Here's the drawing with two shaded views (mm, measured from the low corner). I have some questions. A direction names the side the tool comes from. Give positions to 0.01 mm unless a question says otherwise; leave off trailing zeros. Loops run counter-clockwise (first coordinate to the right, second up) from the corner with the lowest first, then second, coordinate; pieces in that order, holes last. Notation, with made-up numbers: M -16,45 L -10,45 A27 cw -10,71 Z; hole C 76,-1 d5. An arc over 180 degrees is marked long. Use a Markdown table: item, result. Add a question column.
1) Suppose I cut it at D-D on x = 72.5. List the corners of the cut face in (y, z) for me, and give its area (3 significant figures).
2) Suppose I cut it at A-A on z = 2. List the corners of the cut face in (x, y) for me.
3) If I drill on line 1 along Y through (x, z) = (45.5, 3); line 2 along X through (y, z) = (9, 5); line 3 along Y through (x, z) = (74.5, 4.25), over which ranges is the centre line in solid material (lowest first)? Write a range as [from, to].
4) We'd pull the mould along X, two halves only. Please class the marked faces 6, 7, 8 and 9: +X half, -X half, draft (parallel to the pull), parting line (faces both ways), or undercut.
5) Suppose I cut it at B-B on y = 20. List the corners of the cut face in (x, z) for me, and give its area (3 significant figures).
6) Suppose I cut it at C-C on x = 45.5. List the corners of the cut face in (y, z) for me, and give its area (3 significant figures).
7) Will these pins go through, and if not, where does the flat tip stop? pin 1 Ø0.6 at (y, z) = (34.5, 2.5) entering from -X; pin 2 Ø4 at (x, z) = (15, 2) entering from -Y; pin 3 Ø0.6 at (y, z) = (33.5, 4) entering from +X; pin 4 Ø2 at (x, y) = (72, 5.5) entering from +Z.
8) Which directions (+Z, -Z, +X, -X, +Y, -Y) give clear straight access to the entire face, cutting with the end or side of a thin tool? Please do the marked faces 1, 2, 3, 4 and 5.
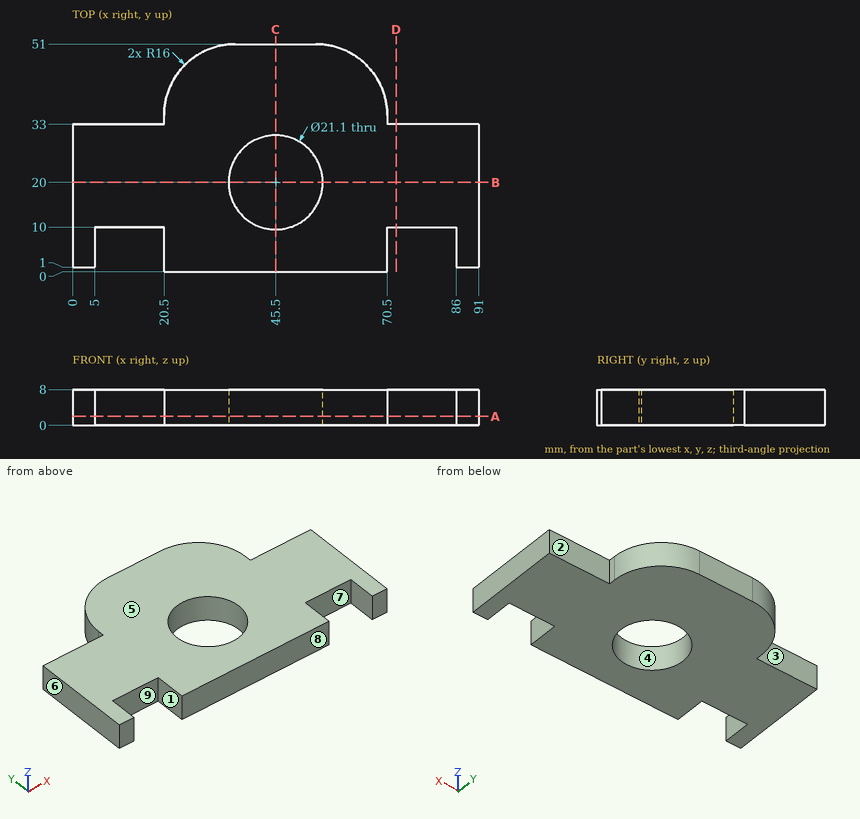
Answer block:
| question | item | result |
|---|---|---|
| 1 | outline | M 10,0 L 33,0 L 33,8 L 10,8 Z |
| 1 | area | 184 mm^2 |
| 2 | outline | M 0,1 L 5,1 L 5,10 L 20.5,10 L 20.5,0 L 70.5,0 L 70.5,10 L 86,10 L 86,1 L 91,1 L 91,33 L 70.5,33 L 70.5,35 A16 ccw 54.5,51 L 36.5,51 A16 ccw 20.5,35 L 20.5,33 L 0,33 Z; hole C 45.5,20 d21.1 |
| 3 | line 1 | y = [0, 9.45], [30.55, 51] |
| 3 | line 2 | x = [0, 5], [20.5, 70.5], [86, 91] |
| 3 | line 3 | y = [10, 33] |
| 4 | face 6 | -X half |
| 4 | face 7 | undercut |
| 4 | face 8 | draft |
| 4 | face 9 | undercut |
| 5 | outline | M 0,0 L 34.95,0 L 34.95,8 L 0,8 Z; M 56.05,0 L 91,0 L 91,8 L 56.05,8 Z |
| 5 | area | 559 mm^2 |
| 6 | outline | M 0,0 L 9.45,0 L 9.45,8 L 0,8 Z; M 30.55,0 L 51,0 L 51,8 L 30.55,8 Z |
| 6 | area | 239 mm^2 |
| 7 | pin 1 | stops at x = 20.5 |
| 7 | pin 2 | stops at y = 10 |
| 7 | pin 3 | stops at x = 70.5 |
| 7 | pin 4 | passes through |
| 8 | face 1 | +Z, -Z, -Y |
| 8 | face 2 | +Z, -Z, +X, +Y |
| 8 | face 3 | +Z, -Z, -X, +Y |
| 8 | face 4 | +Z, -Z |
| 8 | face 5 | +Z, +X, -X, +Y, -Y |
